Verification items for the finished model (mm, model axes). A direction names the side the tool comes from. Coordinates: 2 decimals unless noted, no trailing zeros. Order: outer loops, then holes, each group sorted by start corner. A loop starts at its lowest first (then second) coordinate and runs counter-clockwise, first axis right, second up. Notation, with made-up numbers: (30, 36.5) -> (74, 36.5) arc R26 cw to (74, 61.5) -> close; hole circle Ø3 at (47, -3.75). An arc over 180 degrees is marked (long way). Write item = value, one per line. Start each with the question number.
from build123d import *

# Parameters (mm, degrees)
ESQUISSE1_W             = 40
ESQUISSE1_H             = 120
BOSS_EXTRU_1_DEPTH      = 6
ESQUISSE2_W             = 20
ESQUISSE2_H             = 70
ENL_V_MAT_EXTRU_1_DEPTH = 6
ESQUISSE3_R             = 1.5
ENL_V_MAT_EXTRU_2_DEPTH = 6
ESQUISSE4_R             = 2.995
ENL_V_MAT_EXTRU_3_DEPTH = 3
ESQUISSE6_R             = 1.5
ENL_V_MAT_EXTRU_4_DEPTH = 6


with BuildPart() as part:
    # Esquisse1 → Boss.-Extru.1 (new body)
    with BuildSketch(Plane.XY):
        with Locations((20, 60)):
            Rectangle(ESQUISSE1_W, ESQUISSE1_H)
    extrude(amount=BOSS_EXTRU_1_DEPTH)

    # Esquisse2 → Enlèv. mat.-Extru.1 (cut)
    with BuildSketch(Plane.XY.offset(6)):
        with Locations((30, 85)):
            Rectangle(ESQUISSE2_W, ESQUISSE2_H)
    extrude(amount=-ENL_V_MAT_EXTRU_1_DEPTH, mode=Mode.SUBTRACT)

    # Esquisse3 → Enlèv. mat.-Extru.2 (cut)
    with BuildSketch(Plane.XY.offset(6)):
        with Locations((3, 3)):
            Circle(ESQUISSE3_R)
        with Locations((37, 47)):
            Circle(ESQUISSE3_R)
    extrude(amount=-ENL_V_MAT_EXTRU_2_DEPTH, mode=Mode.SUBTRACT)

    # Esquisse4 → Enlèv. mat.-Extru.3 (cut)
    with BuildSketch(Plane.XY.offset(6)):
        with Locations((3, 3)):
            Circle(ESQUISSE4_R)
        with Locations((37, 47)):
            Circle(ESQUISSE4_R)
    extrude(amount=-ENL_V_MAT_EXTRU_3_DEPTH, mode=Mode.SUBTRACT)

    # Esquisse6 → Enlèv. mat.-Extru.4 (cut)
    with BuildSketch(Plane.XY.offset(6)):
        with Locations((10, 50)):
            Circle(ESQUISSE6_R)
    extrude(amount=-ENL_V_MAT_EXTRU_4_DEPTH, mode=Mode.SUBTRACT)


solid = part.part
Item 1: Tool access check on faces 1 (the flat face through (30, 50, 3)), 2 (the flat face through (40, 25, 3)), 3 (the flat face through (4.3, 1.7, 3)). Record the directions out of +Z, -Z, +X, -X, +Y, -Y that give a thin tool (end or side, any length) a straight path to the whole face; none if there is none.
Item 2: Mould release check, pull along Y, two halves, no side actions. Record for faces 4 (the cylindrical face through (38.61, 49.525, 4.521)), 5 (the cylindrical face through (3.69, 1.67, 1.52)), 6 (the flat face through (20, 85, 3)), 7 (the flat face through (20, 0, 3)): pulls with the +Y half, pulls with the -Y half, needs draft (parallel to the pull), parting line crosses it, or undercut.
Item 3: Thickness scan on line 1 (Y direction, x = 10, z = 3.85); line 2 (Y direction, x = 26.5, z = 0.75); line 3 (X direction, y = 79.5, z = 0.45). Record the ranges inside material, lowest first.
Item 4: Section check C-C (x = 3). Record the boundary of the cut face in (y, z) (3 decimals).
Item 5: Section check A-A (z = 1). Record the boundary of the cut face in (x, y), then the cut area to 3 significant figures.
Item 6: Gauge pin test, flat ends, axial feed: P1, Ø5, axis at x = 35.5, y = 46.5, coming from the +Z side; P2, Ø4, axis at x = 3, y = 3, coming from the +Z side. Record the tip position at first contact, or that the pin passes through.
Item 7: Section check D-D (x = 37). Record the boundary of the cut face in (y, z) (3 decimals).
Item 8: Section check B-B (x = 10). Record the boundary of the cut face in (y, z).
Filled sheet:
q1.face_1 = +Z, -Z, +X, +Y
q1.face_2 = +Z, -Z, +X, +Y, -Y
q1.face_3 = +Z
q2.face_4 = undercut
q2.face_5 = undercut
q2.face_6 = needs draft
q2.face_7 = pulls with the -Y half
q3.line_1 = 0 to 48.5, 51.5 to 120
q3.line_2 = 0 to 50
q3.line_3 = 0 to 20
q4.outline = (0, 0) -> (1.5, 0) -> (1.5, 3) -> (0.005, 3) -> (0.005, 6) -> (0, 6) -> close; (4.5, 0) -> (120, 0) -> (120, 6) -> (5.995, 6) -> (5.995, 3) -> (4.5, 3) -> close
q5.outline = (0, 0) -> (40, 0) -> (40, 50) -> (20, 50) -> (20, 120) -> (0, 120) -> close; hole circle Ø3 at (3, 3); hole circle Ø3 at (10, 50); hole circle Ø3 at (37, 47)
q5.area = 3,380 mm^2
q6.P1 = 6
q6.P2 = 3
q7.outline = (0, 0) -> (45.5, 0) -> (45.5, 3) -> (44.005, 3) -> (44.005, 6) -> (0, 6) -> close; (48.5, 0) -> (50, 0) -> (50, 6) -> (49.995, 6) -> (49.995, 3) -> (48.5, 3) -> close
q8.outline = (0, 0) -> (48.5, 0) -> (48.5, 6) -> (0, 6) -> close; (51.5, 0) -> (120, 0) -> (120, 6) -> (51.5, 6) -> close
